from build123d import *
from build123d.topology import SkipClean

# Parameters (mm, degrees)
SKETCH1_R                  = 157.48000000000002
EXTRUDE1_DEPTH             = 70.10399999999998
SKETCH2_R                  = 47.0535
EXTRUDE2_DEPTH             = 24.130000000000003
SKETCH3_R                  = 15.011400000000002
EXTRUDE3_DEPTH             = 13.462
SKETCH4_R                  = 24.511
EXTRUDE4_DEPTH             = 6.35
SKETCH5_R                  = 15.875
EXTRUDE5_DEPTH             = 6.8580000000000005
SKETCH6_R                  = 3.174999999999999
CUT_EXTRUDE1_DEPTH         = 11.43
CIRPATTERN1_COUNT          = 5
SKETCH7_R                  = 60.325
EXTRUDE6_DEPTH             = 13.970000000000011
CHAMFER1_SIZE              = 10.16
CHAMFER2_SIZE              = 12.7
EXTRUDE7_REACH             = 396.95
EXTRUDE7_END_RADIUS        = 157.48000000000002
SKETCH8_R                  = 19.05
EXTRUDE7_DIRECTION_2_DEPTH = 44.449999999999996


with BuildPart() as part:
    # Sketch1 → Extrude1 (new body)
    with BuildSketch(Plane.XY):
        Circle(SKETCH1_R)
    extrude(amount=EXTRUDE1_DEPTH)

    # Sketch2 → Extrude2 (add)
    with BuildSketch(Plane.XY.offset(70.10399999999998)):
        Circle(SKETCH2_R)
    extrude(amount=EXTRUDE2_DEPTH)

    # Sketch3 → Extrude3 (add)
    with BuildSketch(Plane(origin=(0, 0, 0), x_dir=(-1, 0, 0), z_dir=(0, 0, -1))):
        with Locations(Location((0, 0, 0), (0, 0, 180))):
            Circle(SKETCH3_R)
    extrude(amount=EXTRUDE3_DEPTH)

    # Sketch4 → Extrude4 (add)
    with BuildSketch(Plane(origin=(0, 0, -13.462), x_dir=(-1, 0, 0), z_dir=(0, 0, -1))):
        Circle(SKETCH4_R)
    extrude(amount=EXTRUDE4_DEPTH)

    # Sketch5 → Extrude5 (add)
    with BuildSketch(Plane(origin=(0, 0, -19.812), x_dir=(-1, 0, 0), z_dir=(0, 0, -1))):
        Circle(SKETCH5_R)
    extrude(amount=EXTRUDE5_DEPTH)

    # Sketch6 → Cut-Extrude1 (cut)
    with BuildSketch(Plane(origin=(0, 0, 0), x_dir=(-1, 0, 0), z_dir=(0, 0, -1))):
        with Locations((0, -38.1)):
            Circle(SKETCH6_R)
    cut_extrude1 = extrude(amount=-CUT_EXTRUDE1_DEPTH, mode=Mode.SUBTRACT)

    # CirPattern1: Cut-Extrude1 ×5 about axis
    cirpattern1_axis = Axis((-1.12e-15, 1.2e-15, 0), (0, 0, 1))
    for i in range(1, CIRPATTERN1_COUNT):
        add(cut_extrude1.rotate(cirpattern1_axis, i * 360 / CIRPATTERN1_COUNT), mode=Mode.SUBTRACT)

    # Sketch7 → Extrude6 (add)
    with BuildSketch(Plane.XY.offset(94.23399999999998)):
        with Locations(Location((0, 0, 0), (0, 0, 180))):
            Circle(SKETCH7_R)
    extrude(amount=EXTRUDE6_DEPTH)

    # Chamfer1
    chamfer1_edges = [part.edges().sort_by_distance(p)[0] for p in [
        (-157.48000000000002, 1.929e-14, 0),
        (-157.48000000000002, 1.929e-14, 70.10399999999998),
    ]]
    chamfer(chamfer1_edges, length=CHAMFER1_SIZE)

    # Chamfer2
    chamfer2_edges = [part.edges().sort_by_distance(p)[0] for p in [
        (60.325, -1.478e-14, 108.204),
    ]]
    chamfer(chamfer2_edges, length=CHAMFER2_SIZE)

    # Extrude7: up to this cylinder (the profile starts outside it)
    with SkipClean():  # the faces are left unmerged after this step: merging them gives an invalid solid
        extrude7_end = Plane(origin=(0, 0, 34.29), z_dir=(0, 0, -1)) * Cylinder(EXTRUDE7_END_RADIUS, 1109.8600000000001, mode=Mode.PRIVATE)
        # Sketch8 → Extrude7 (add, up to the surface)
        with BuildSketch(Plane(origin=(-101.22619277343593, 120.63667890237693, 0), x_dir=(0.7660444431189796, 0.6427876096865376, 0), z_dir=(0.6427876096865376, -0.7660444431189797, 0)), mode=Mode.PRIVATE) as extrude7_sk1:
            with Locations(Location((-1.388e-14, 34.290000000000056, 0), (0, 0, 180))):
                Circle(SKETCH8_R)
        extrude7_tool1 = extrude(extrude7_sk1.sketch, amount=EXTRUDE7_REACH, mode=Mode.PRIVATE) - extrude7_end
        add(extrude7_tool1.solids().sort_by_distance((-101.226193, 120.636679, 34.29))[0])
        add(extrude7_tool1.solids().sort_by_distance((-101.226193, 120.636679, 34.29))[1])

    # Sketch8 → Extrude7 direction 2 (add)
    with BuildSketch(Plane(origin=(-101.22619277343593, 120.63667890237693, 0), x_dir=(0.7660444431189796, 0.6427876096865376, 0), z_dir=(0.6427876096865376, -0.7660444431189797, 0))):
        with Locations(Location((-1.388e-14, 34.290000000000056, 0), (0, 0, 180))):
            Circle(SKETCH8_R)
    extrude(amount=-EXTRUDE7_DIRECTION_2_DEPTH)


solid = part.part
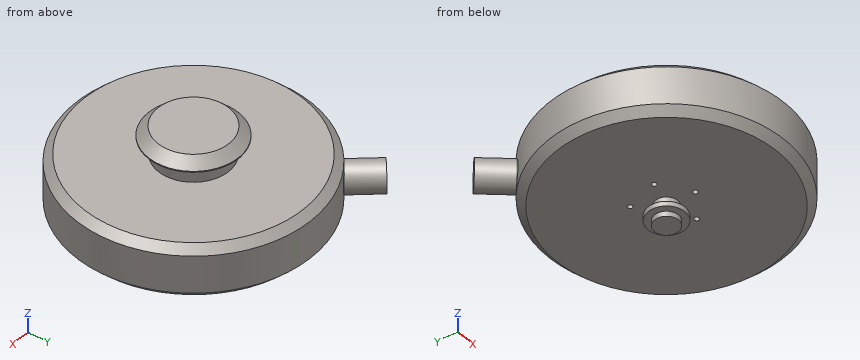
Verification items for the finished model (mm, model axes). Coordinates: 2 decimals unless noted, no trailing zeros. Order: outer loops, then holes, each group sorted by start corner. A loop starts at its lowest first (then second) coordinate and runs counter-clockwise, first axis right, second up. Notation, with made-up numbers: M -1.5,25 L 2.5,25 A14 ccw 2.5,32 Z; hole C 67,-22.5 d10. An arc over 180 degrees is marked long. One line per item, written item: value. Start each with the question number.
Item 1: Scan lines: probe 1 along Z at (x, y) = (113.5, -91); probe 2 along Y at (x, z) = (0, 3.25) (3 decimals); probe 3 along Z at (x, y) = (-50.5, 15). Record each from-to range of solid material in increasing order.
Item 2: Sectioned sample at B-B (z = 80). Enter the section's corners in (x, y).
Item 3: Sectioned sample at C-C (z = 30.5). Enter the section's corners in (x, y).
Item 4: Gauge pin test, flat ends, axial feed: pin 1 (1 mm diameter, centred on x = -65.5, z = -1.5, fed in from +Y); pin 2 (1 mm diameter, centred on x = 85, y = -106, fed in from +Z); pin 3 (3 mm diameter, centred on x = -1, y = -37, fed in from -Z); pin 4 (10 mm diameter, centred on x = 95.5, y = 80, fed in from -Z). Record the tip position at first contact, or that the pin passes through.
Conclusion:
1. probe 1: z = 0 to 70.1
1. probe 2: y = -150.57 to -41.275, -34.925 to 150.57
1. probe 3: z = 0 to 70.1, 94.23 to 103.15
2. outline: C 0,0 d94.11
3. outline: M -144.1,142.69 L -114.81,107.79 A157.48 ccw long -86.21,131.79 L -115.5,166.69 Z
4. pin 1: passes through
4. pin 2: stops at z = 70.1
4. pin 3: stops at z = 11.43
4. pin 4: stops at z = 0
